Autodesk Inventor part; units mm, degrees
ref_plane "YZ Plane" through (0, 0, 0) normal (1, 0, 0) x (0, 1, 0)
ref_plane "XZ Plane" through (0, 0, 0) normal (0, 1, 0) x (-1, 0, 0)
ref_plane "XY Plane" through (0, 0, 0) normal (0, 0, 1) x (1, 0, 0)
sketch "Sketch1" plane through (0, 0, 0) normal (1, 0, 0) x (0, 1, 0)
  arc A0 (-13.4131, 0) -> (13.4131, 0) centre (0, 0) ccw
  arc A1 (-15.9131, 0) -> (15.9131, 0) centre (0, 0) ccw
  arc A2 (13.4131, 63.0094) -> (-13.4131, 63.0094) centre (0, 63.0094) ccw
  arc A3 (15.9131, 63.0094) -> (-15.9131, 63.0094) centre (0, 63.0094) ccw
  line L0 (13.4131, 0) -> (13.4131, 63.0094)
  line L1 (-13.4131, 0) -> (-13.4131, 63.0094)
  line L2 (15.9131, 0) -> (15.9131, 63.0094)
  line L3 (-15.9131, 0) -> (-15.9131, 63.0094)
  dimension "d0" = 2.5
  dimension "d1" = 13.4131
  dimension "d2" = 63.0094
extrude "Extrusion1" add sketch "Sketch1" along normal blind 9
properties part number "STANDIN,130T,HTD5mm,BELT" material "Nylon 6/6"
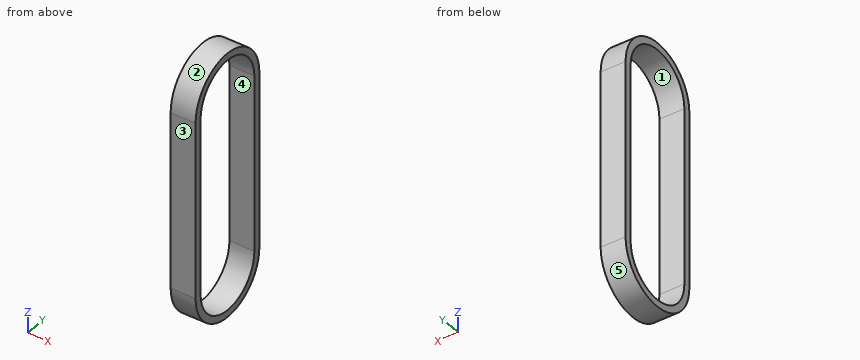
Geometry check sheet. Reference: the model listing, model coordinates, mm. Face numbers are marked on the shaded views. A direction names the side the tool comes from. Give positions to 0.01 mm unless a question says otherwise; leave off trailing zeros. Loops run counter-clockwise (first coordinate to the right, second up) from the corner with the lowest first, then second, coordinate; pieces in that order, holes last.
(1) Release check for a two-part mould opening along Z. For the marked faces 3, 4 and 5 record: released by +Z, released by -Z, zero draft, split by the parting line, or undercut.
From the geometry:
face 3: zero draft
face 4: undercut
face 5: released by -Z
(2) Section check A-A on x = 5.75. Record the cut outline in (y, z), then the cut area to 3 significant figures.
From the geometry:
outline: (-15.91, 0) arc R15.91 ccw to (15.91, 0) - (15.91, 63.01) arc R15.91 ccw to (-15.91, 63.01) - close; hole (-13.41, 0) arc R13.41 ccw to (13.41, 0) - (13.41, 63.01) arc R13.41 ccw to (-13.41, 63.01) - close
area: 545 mm2
(3) Set-up check for the marked faces 1 and 2: record each of +Z, -Z, +X, -X, +Y, -Y from which the full face is reachable in a straight line by a thin tool's end or side.
From the geometry:
face 1: +X, -X
face 2: +Z, +X, -X
(4) Section check C-C on y = 0. Record the cut outline in (x, z).
From the geometry:
outline: (0, -15.91) - (9, -15.91) - (9, -13.41) - (0, -13.41) - close; (0, 76.42) - (9, 76.42) - (9, 78.92) - (0, 78.92) - close
(5) Depth check by flat-ended pin: pin 1 Ø1 at (x, y) = (1, 5) entering from +Z; pin 2 Ø6 at (y, z) = (7.5, 39.5) entering from +X; pin 3 Ø3 at (x, z) = (1, 66) entering from +Y. Enter the tip coordinate at first touch or a pass-through.
From the geometry:
pin 1: stops at z = 78.27
pin 2: passes through
pin 3: stops at y = 15.84
(6) Thickness scan on L1, parallel to Z at x = 3.75, y = 0; L2, parallel to Y at x = 5.25, z = 39; L3, parallel to Z at x = 7.5, y = -10.5. Record the ranges inside material, lowest first.
From the geometry:
L1: z = -15.91 to -13.41, 76.42 to 78.92
L2: y = -15.91 to -13.41, 13.41 to 15.91
L3: z = -11.96 to -8.35, 71.36 to 74.97
(7) Section check B-B on z = 13. Record the cut outline in (x, y), then the cut area to 3 significant figures.
From the geometry:
outline: (0, -15.91) - (9, -15.91) - (9, -13.41) - (0, -13.41) - close; (0, 13.41) - (9, 13.41) - (9, 15.91) - (0, 15.91) - close
area: 45.0 mm2
